from build123d import *

# Parameters (mm, degrees)
F_4_CLEARANCE_HOLE1_D     = 2.9464
F_4_CLEARANCE_HOLE1_DEPTH = 38.354
F_4_CLEARANCE_HOLE1_TIP   = 0.885187864


with BuildPart() as part:
    # Sketch1 → Revolve1 (revolve)
    with BuildSketch(Plane.XY, mode=Mode.PRIVATE) as revolve1_sk:
        with BuildLine():
            Line((5.55625, 0), (5.55625, 12.019409051))
            ThreePointArc((5.55625, 12.019409051), (5.772621003, 13.662909988), (6.406988686, 15.194409051))
            Line((6.406988686, 15.194409051), (24.549261314, 46.617747008))
            ThreePointArc((24.549261314, 46.617747008), (25.183628997, 48.149246071), (25.4, 49.792747008))
            Line((25.4, 49.792747008), (25.4, 53.34))
            Line((25.4, 53.34), (27.94, 53.34))
            Line((27.94, 53.34), (27.94, 52.29225))
            ThreePointArc((27.94, 52.29225), (28.098089115, 51.910589115), (28.47975, 51.7525))
            Line((28.47975, 51.7525), (28.98775, 51.7525))
            ThreePointArc((28.98775, 51.7525), (29.369410885, 51.910589115), (29.5275, 52.29225))
            Line((29.5275, 52.29225), (29.5275, 53.34))
            Line((29.5275, 53.34), (38.983295256, 53.34))
            Line((38.983295256, 53.34), (38.983295256, 50.8))
            Line((38.983295256, 50.8), (33.196382361, 50.8))
            ThreePointArc((33.196382361, 50.8), (31.608882361, 50.374630657), (30.446751704, 49.2125))
            Line((30.446751704, 49.2125), (10.216988686, 14.173522628))
            ThreePointArc((10.216988686, 14.173522628), (9.582621003, 12.642023564), (9.36625, 10.998522628))
            Line((9.36625, 10.998522628), (9.36625, 0))
            Line((9.36625, 0), (5.55625, 0))
        make_face()
    revolve(revolve1_sk.sketch.rotate(Axis((0, 0, 0), (0, 1, 0)), 90), axis=Axis((0, 0, 0), (0, 1, 0)))

    # #4 Clearance Hole1
    with Locations(Plane(origin=(0, 50.8, 0), x_dir=(-1, 0, 0), z_dir=(0, -1, 0))):
        with Locations((35.56, 0), (25.144717139, -25.144717139), (0, -35.56), (-25.144717139, -25.144717139), (-35.56, 0), (-25.144717139, 25.144717139), (0, 35.56), (25.144717139, 25.144717139), (0, 0)):
            Hole(F_4_CLEARANCE_HOLE1_D / 2, depth=F_4_CLEARANCE_HOLE1_DEPTH)
            with Locations((0, 0, -(F_4_CLEARANCE_HOLE1_DEPTH + F_4_CLEARANCE_HOLE1_TIP / 2))):  # 118° drill point
                Cone(0, F_4_CLEARANCE_HOLE1_D / 2, F_4_CLEARANCE_HOLE1_TIP, mode=Mode.SUBTRACT)


solid = part.part
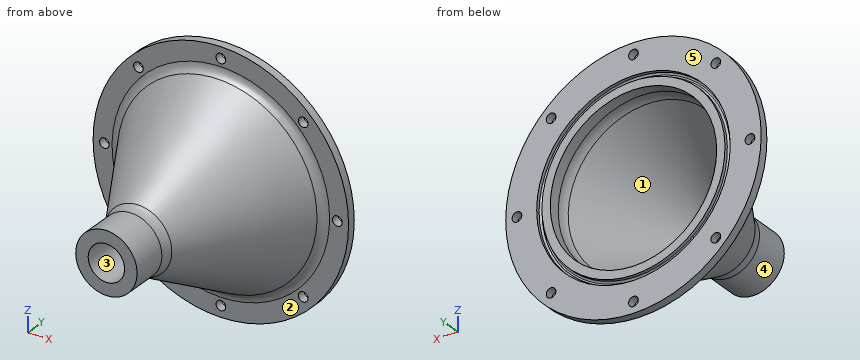
Here's how the part is built. I have some questions about the finished solid (model axes, mm). Face numbers are marked on the shaded views. A direction names the side the tool comes from. Coordinates: 2 decimals unless noted, no trailing zeros. Write each loop counter-clockwise with the first axis right and the second up, starting at its lowest first coordinate (ties: lowest second). Pieces come first, ordered by that corner, then holes.
Item 1: I want a section at C-C on y = 8. Write out the boundary of the cut face in (x, z).
Item 2: I want a section at A-A on x = 35.56. Write out the boundary of the cut face in (y, z), and give its area (3 significant figures).
Item 3: If I drill on line 1 (Z direction, x = -20, y = 43); line 2 (Y direction, x = -35, z = -13); line 3 (X direction, y = 17.5, z = -6.5), over which ranges is the centre line in solid material (lowest first)?
Item 4: I want a section at B-B on z = -35.56. Write out the boundary of the cut face in (x, y).
Item 5: Will these pins go through, and if not, where does the flat tip stop? pin 1 (10 mm diameter, centred on x = -4, y = 14.5, fed in from -Z); pin 2 (4.5 mm diameter, centred on x = -35.56, z = 0, fed in from -Y); pin 3 (6 mm diameter, centred on y = 22.5, z = -9.5, fed in from +X).
Item 6: I want a section at D-D on x = 0. Count the separate pieces of the cut face and the enclosed holes in it, and give its area (3 significant figures).
Item 7: On a 3-axis mill with a long thin cutter (end or side, diameter ignored), from which of +Z, -Z, +X, -X, +Y, -Y can I reach the whole of each face in a straight line? I mean the marked faces 1 and 2. Say none if no direction works.
Item 8: If we mould it in two halves opening along X, with no side actions, what happens to the marked faces 3, 4 and 5? For each: +X half, -X half, draft (parallel to the pull), parting line (faces both ways), or undercut.
Findings below:
1. outline: circle Ø18.73 at (0, 0); hole circle Ø11.11 at (0, 0)
2. outline: (50.8, -15.97) - (53.34, -15.97) - (53.34, -1.47) - (50.8, -1.47) - close; (50.8, 1.47) - (53.34, 1.47) - (53.34, 15.97) - (50.8, 15.97) - close
2. area: 73.7 mm2
3. line 1: z = -17.93 to -10.22, 10.22 to 17.93
3. line 2: y = 50.8 to 53.34
3. line 3: x = -10.25 to -4.2, 4.2 to 10.25
4. outline: (-15.97, 50.8) - (-1.47, 50.8) - (-1.47, 53.34) - (-15.97, 53.34) - close; (1.47, 50.8) - (15.97, 50.8) - (15.97, 53.34) - (1.47, 53.34) - close
5. pin 1: stops at z = -12.92
5. pin 2: stops at y = 50.8
5. pin 3: stops at x = 14.49
6. separate pieces: 4
6. enclosed holes: 0
6. area: 486 mm2
7. face 1: +Y
7. face 2: -Y
8. face 3: undercut
8. face 4: parting line
8. face 5: draft
